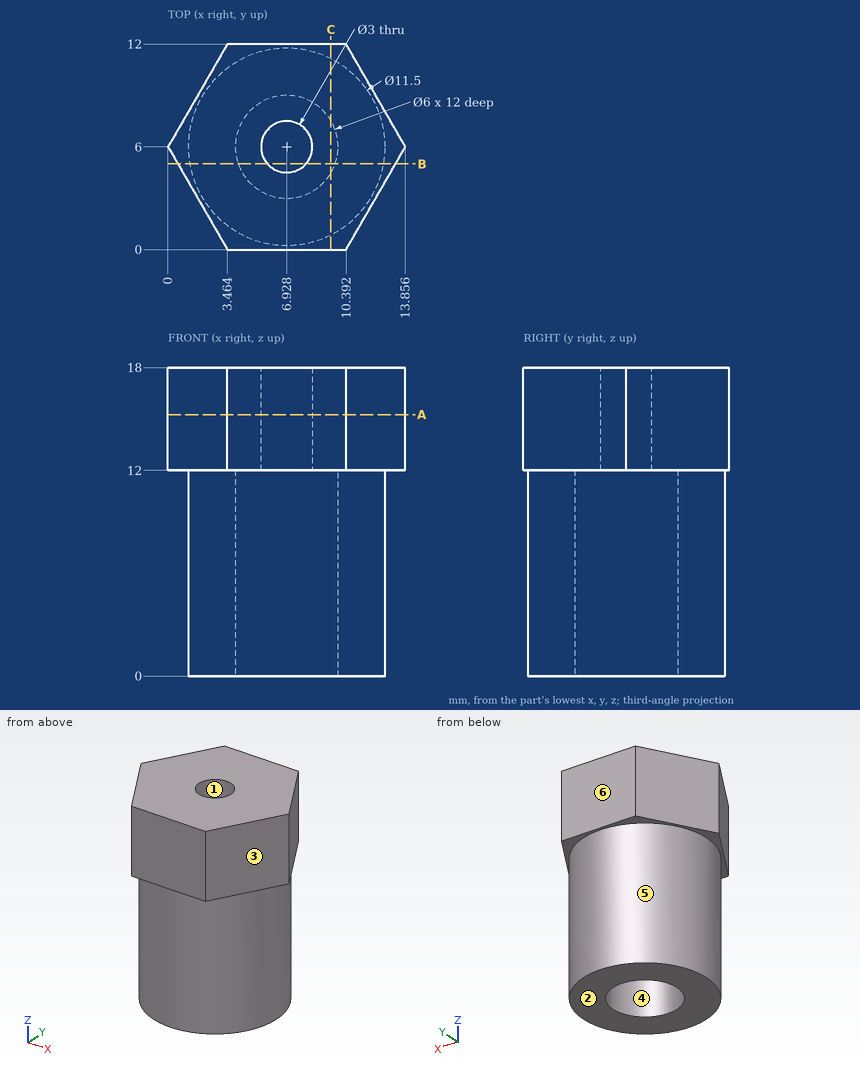
Geometry check sheet. Reference: drawing and pictorial views, mm from the part's lowest x, y, z. A direction names the side the tool comes from. Round coordinates to 2 decimals unless told otherwise and drop trailing zeros. Loops run counter-clockwise (first coordinate to the right, second up) from the corner with the lowest first, then second, coordinate; pieces in that order, holes last. Notation, with made-up numbers: (40.25, -37) - (71.25, -37) arc R25 ccw to (71.25, -9) - close; hole circle Ø1 at (-29, -15.5). An arc over 180 degrees is marked (long way). Use a Markdown table: item, result. Add a question column.
1. Gauge pin test, flat ends, axial feed: pin 1 (5.5 mm diameter, centred on x = 6.93, y = 6, fed in from -Z); pin 2 (1 mm diameter, centred on x = 11.5, z = 4, fed in from -Y); pin 3 (1.8 mm diameter, centred on x = 6.93, y = 6, fed in from -Z); pin 4 (5 mm diameter, centred on x = 5, z = 2, fed in from -Y). Record the tip position at first contact, or that the pin passes through.
2. Section check B-B, the plane y = 5. Record the boundary of the cut face in (x, z).
3. Section check C-C, the plane x = 9.5. Record the boundary of the cut face in (y, z) (1 decimal).
4. Section check A-A, the plane z = 15.25. Record the boundary of the cut face in (x, y).
5. Release check for a two-part mould opening along Y. For the marked faces 1, 2, 3 and 4 record: released by +Y, released by -Y, zero draft, split by the parting line, or undercut.
6. Thickness scan on probe 1 along Z at (x, y) = (5, 7); probe 2 along Y at (x, z) = (5.25, 8) (1 decimal); probe 3 along Y at (x, z) = (3.25, 15.5). Record the ranges inside material, lowest first. Write a range as [from, to].
7. Access from +Z, -Z, +X, -X, +Y, -Y to the whole of each face (thin tool, end or side, straight path). Record for the marked faces 5 and 6.
Checks:
| question | item | result |
|---|---|---|
| 1 | pin 1 | stops at z = 12 |
| 1 | pin 2 | stops at y = 1.94 |
| 1 | pin 3 | passes through |
| 1 | pin 4 | stops at y = 0.25 |
| 2 | outline | (0.58, 12) - (1.27, 12) - (1.27, 0) - (4.1, 0) - (4.1, 12) - (5.81, 12) - (5.81, 18) - (0.58, 18) - close; (8.05, 12) - (9.76, 12) - (9.76, 0) - (12.59, 0) - (12.59, 12) - (13.28, 12) - (13.28, 18) - (8.05, 18) - close |
| 3 | outline | (0, 12) - (0.9, 12) - (0.9, 0) - (4.5, 0) - (4.5, 12) - (7.5, 12) - (7.5, 0) - (11.1, 0) - (11.1, 12) - (12, 12) - (12, 18) - (0, 18) - close |
| 4 | outline | (0, 6) - (3.46, 0) - (10.39, 0) - (13.86, 6) - (10.39, 12) - (3.46, 12) - close; hole circle Ø3 at (6.93, 6) |
| 5 | face 1 | undercut |
| 5 | face 2 | zero draft |
| 5 | face 3 | released by -Y |
| 5 | face 4 | undercut |
| 6 | probe 1 | z = [12, 18] |
| 6 | probe 2 | y = [0.5, 3.5], [8.5, 11.5] |
| 6 | probe 3 | y = [0.37, 11.63] |
| 7 | face 5 | -Z |
| 7 | face 6 | +Z, -Z, +X, -X, +Y |
